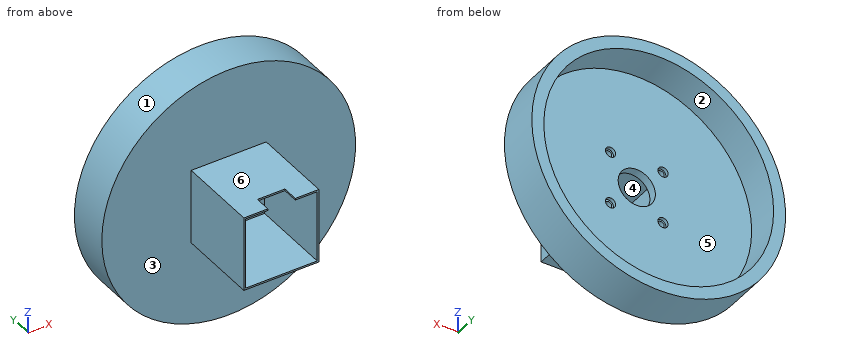
Autodesk Inventor part; units mm, degrees
ref_plane "YZ Plane" through (0, 0, 0) normal (1, 0, 0) x (0, 1, 0)
ref_plane "XZ Plane" through (0, 0, 0) normal (0, 1, 0) x (-1, 0, 0)
ref_plane "XY Plane" through (0, 0, 0) normal (0, 0, 1) x (1, 0, 0)
sketch "Эскиз1" plane through (0, 0, 0) normal (0, 1, 0) x (-1, 0, 0)
  circle A0 centre (0, 0) radius 75
  dimension "d0" = 150
extrude "Выдавливание1" add sketch "Эскиз1" along normal blind 5
sketch "Эскиз2" plane through (0, 0, 0) normal (0, -1, 0) x (1, 0, 0)
  line L0 (21.175, 21.175) -> (-21.175, 21.175)
  line L1 (-21.175, 21.175) -> (-21.175, -21.175)
  line L2 (-21.175, -21.175) -> (21.175, -21.175)
  line L3 (21.175, -21.175) -> (21.175, 21.175)
  line L4 (21.175, 21.175) -> (-21.175, -21.175) construction
  line L5 (-21.175, 21.175) -> (21.175, -21.175) construction
  line L6 (22.175, 22.175) -> (-22.175, 22.175)
  line L7 (-22.175, 22.175) -> (-22.175, -22.175)
  line L8 (-22.175, -22.175) -> (22.175, -22.175)
  line L9 (22.175, -22.175) -> (22.175, 22.175)
  line L10 (22.175, 22.175) -> (-22.175, -22.175) construction
  line L11 (-22.175, 22.175) -> (22.175, -22.175) construction
  point P0 (0, 0)
  dimension "d3" = 42.35
  dimension "d4" = 42.35
  dimension "d5" = 44.35
  dimension "d6" = 44.35
extrude "Выдавливание2" add sketch "Эскиз2" along normal blind 48
sketch "Эскиз4" plane through (-22.175, 0, 22.175) normal (0, 0, 1) x (1, 0, 0)
  line L0 (0, 0) -> (0, -48)
  line L1 (22.175, -48) -> (30.425, -48)
  line L2 (30.425, -48) -> (30.425, -38.5)
  line L3 (30.425, -38.5) -> (14.175, -38.5)
  line L4 (14.175, -38.5) -> (14.175, -48)
  line L5 (22.175, -48) -> (14.175, -48)
  point P0 (22.175, 0)
  dimension "d9" = 22.175
  dimension "d10" = 8.25
  dimension "d11" = 9.5
  dimension "d12" = 16.25
extrude "Выдавливание3" cut sketch "Эскиз4" against normal blind 1
sketch "Эскиз5" plane through (0, 5, 0) normal (0, 1, 0) x (1, 0, 0)
  circle A0 centre (0, 0) radius 11
  line L0 (-15.5, -15.5) -> (15.5, -15.5)
  line L1 (15.5, -15.5) -> (15.5, 15.5)
  line L2 (15.5, 15.5) -> (-15.5, 15.5)
  line L3 (-15.5, 15.5) -> (-15.5, -15.5)
  line L4 (-15.5, -15.5) -> (15.5, 15.5) construction
  line L5 (15.5, -15.5) -> (-15.5, 15.5) construction
  circle A1 centre (15.5, 15.5) radius 2
  circle A2 centre (15.5, -15.5) radius 2
  circle A3 centre (-15.5, -15.5) radius 2
  circle A4 centre (-15.5, 15.5) radius 2
  dimension "d15" = 22
  dimension "d16" = 31
  dimension "d17" = 31
  dimension "d18" = 4
  dimension "d19" = 4
  dimension "d20" = 4
  dimension "d21" = 4
extrude "Выдавливание4" cut sketch "Эскиз5" against normal blind 5 contours A0 | L3 A3 L0 | L0 A3 L3 | A2 L1 L0 | L0 L1 A2 | A4 L2 L3 | L3 L2 A4 | A1 L2 L1 | L1 L2 A1
sketch "Эскиз6" plane through (0, 5, 0) normal (0, 1, 0) x (1, 0, 0)
  circle A0 centre (15.5, 15.5) radius 2
  line L0 (-15.5, -15.5) -> (15.5, -15.5)
  line L1 (15.5, -15.5) -> (15.5, 15.5)
  line L2 (15.5, 15.5) -> (-15.5, 15.5)
  line L3 (-15.5, 15.5) -> (-15.5, -15.5)
  line L4 (-15.5, -15.5) -> (15.5, 15.5) construction
  line L5 (15.5, -15.5) -> (-15.5, 15.5) construction
  circle A1 centre (15.5, 15.5) radius 3
  circle A2 centre (15.5, -15.5) radius 3
  circle A3 centre (-15.5, -15.5) radius 2
  circle A4 centre (-15.5, -15.5) radius 3
  circle A5 centre (-15.5, 15.5) radius 2
  circle A6 centre (-15.5, 15.5) radius 3
  point P0 (0, 0)
  dimension "d24" = 6
  dimension "d25" = 6
  dimension "d26" = 6
  dimension "d27" = 6
extrude "Выдавливание5" cut sketch "Эскиз6" against normal blind 2 contours A0 L1 L2 | A0 L2 A1 L1 | L2 L1 A0 | A0 L1 A1 L2 | A6 L3 A5 L2 | L2 A5 L3 A6 | A2 L0 L1 | L1 L0 A2 | A5 L3 L2 | L2 L3 A5 | A4 L0 A3 L3 | L3 A3 L0 A4 | A3 L0 L3 | L3 L0 A3
sketch "Эскиз7" plane through (0, 5, 0) normal (0, 1, 0) x (1, 0, 0)
  circle A0 centre (0, 0) radius 67.9085
  circle A1 centre (0, 0) radius 75
  dimension "d30" = 135.817
  dimension "d31" = 150
extrude "Выдавливание6" add sketch "Эскиз7" along normal blind 20
properties part number "Основание"
Could you check a few things on this model? Use its own coordinates, in mm. Face numbers are marked on the shaded views. A direction names the side the tool comes from. Coordinates: 2 decimals unless noted, no trailing zeros. Loops run counter-clockwise (first coordinate to the right, second up) from the corner with the lowest first, then second, coordinate; pieces in that order, holes last. Notation, with made-up numbers: M 54,80.25 L 79,80.25 A14 ccw 79,97.25 Z; hole C 61,-28.5 d2. An arc over 180 degrees is marked long. Put each result on its own line as item: value. Start each with the question number.
(1) Thinking about a two-plate mould opening in X: for the marked faces 1, 2 and 3, which applies, pulls with the +X half, pulls with the -X half, needs draft (parallel to the pull), parting line crosses it, or undercut?
(2) Will these pins go through, and if not, where does the flat tip stop? P1, Ø12, axis at x = -28, z = 7.5, coming from the +Y side; P2, Ø8, axis at y = -13, z = 19.5, coming from the -X side (3 decimals); P3, Ø12.5, axis at x = -2.5, y = -23.5, coming from the -Z side (3 decimals).
(3) Suppose I cut it at B-B on z = 0. Please give me the cut outline in (x, y) (1 decimal), then the cut area to 3 significant figures.
(4) Suppose I cut it at C-C on x = -15.5. Count the separate pieces of the cut face and the enclosed holes in it, then the cut area to 3 significant figures.
(5) I need wall thicknesses on line 1 (Z direction, x = -8, y = -0.5) (3 decimals); line 2 (Z direction, x = 15.5, y = 1.8). Which ranges of each line are inside material? Lowest first, please. Write a range as from..to.
(6) For the marked faces 4, 5 and 6, which set-ups out of +Z, -Z, +X, -X, +Y, -Y let a thin tool reach every point of the face, with its end or its side?
(7) Suppose I cut it at A-A on y = -9. Please give me the cut outline in (x, z) (3 decimals), then the cut area to 3 significant figures.
Solutions:
1. face 1: parting line crosses it
1. face 2: undercut
1. face 3: needs draft
2. P1: stops at y = 5
2. P2: stops at x = -22.175
2. P3: stops at z = -22.175
3. outline: M -75,0 L -22.2,0 L -22.2,-48 L -21.2,-48 L -21.2,0 L -11,0 L -11,5 L -67.9,5 L -67.9,25 L -75,25 Z; M 11,0 L 21.2,0 L 21.2,-48 L 22.2,-48 L 22.2,0 L 75,0 L 75,25 L 67.9,25 L 67.9,5 L 11,5 Z
3. area: 1,020 mm2
4. separate pieces: 3
4. enclosed holes: 0
4. area: 1,070 mm2
5. line 1: z = -22.175..-21.175, 21.175..22.175
5. line 2: z = -73.38..-17.5, -13.5..13.5, 17.5..73.38
6. face 4: -Y
6. face 5: +Y
6. face 6: +Z, +X, -X, -Y
7. outline: M -22.175,-22.175 L 22.175,-22.175 L 22.175,22.175 L -22.175,22.175 Z; hole M -21.175,-21.175 L 21.175,-21.175 L 21.175,21.175 L -21.175,21.175 Z
7. area: 173 mm2
